Source: CAD feature listing. Evaluate the final solid. Frame: model axes, mm. Face numbers are marked on the shaded views. A direction names the side the tool comes from. Give positions to 0.01 mm unless a question says otherwise; leave off trailing zeros. Order: outer loops, then holes, each group sorted by start corner. A loop starts at its lowest first (then second) coordinate and runs counter-clockwise, first axis right, second up.
1) Section B-B, the plane z = -2.5. Return loops of the section in (x, y), plus the area to 3 significant figures.
2) Draft query along Z for the marked faces 1, 2 and 3. Return one class per face: released by +Z, released by -Z, zero draft, split by the parting line, or undercut.
3) Section D-D, the plane x = 27.5. Return loops of the section in (y, z).
4) First-contact query: P1, Ø2, axis at x = 79.5, z = -9, coming from the +Y side; P2, Ø8.5, axis at x = 86, z = -63.5, coming from the +Y side; P3, Ø5, axis at x = 48, y = 6, coming from the +Z side; P4, Ø2.5, axis at x = 2.5, z = -2.5, coming from the -Y side. Flat tips, straight axial feed; report the tip coordinate or a pass-through.
5) Material intervals for line 1 (Z direction, x = 2.5, y = 0.55); line 2 (X direction, y = 7.25, z = 7); line 3 (Z direction, x = 97.5, y = 1.15), sorted ascending.
6) Access query for the marked faces 4, 5, 6, 7 and 8. Directions: +Z, -Z, +X, -X, +Y, -Y. A direction counts if a zero-diameter tool reaches every point of the face in a straight line with its end or side. Return the directions, or none.
7) Section C-C, the plane z = -75. Return loops of the section in (x, y), plus the area to 3 significant figures.
8) Section A-A, the plane x = 55. Return loops of the section in (y, z), plus the area to 3 significant figures.
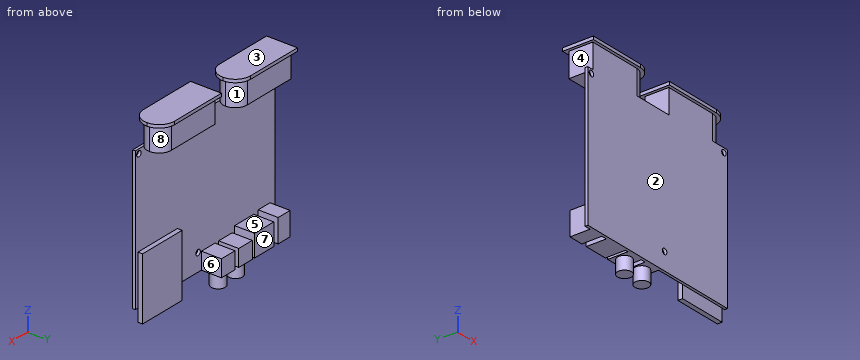
```python
from build123d import *

# Parameters (mm, degrees)
SKETCH1_W            = 100
SKETCH1_H            = 81
BOSS_EXTRUDE1_DEPTH  = 1.6
SKETCH2_W            = 38.5
SKETCH2_H            = 13.8
BOSS_EXTRUDE2_DEPTH  = 14
SKETCH3_W            = 42.4
SKETCH3_H            = 17.7
BOSS_EXTRUDE3_DEPTH  = 1.8
SKETCH4_W            = 8.5
SKETCH4_H            = 13.5
SKETCH4_W_2          = 13.7
SKETCH4_H_2          = 12.6
SKETCH4_W_3          = 9.7
SKETCH4_H_3          = 9.7
BOSS_EXTRUDE4_DEPTH  = 11.5
SKETCH5_W            = 28.3
SKETCH5_H            = 35.8
BOSS_EXTRUDE5_DEPTH  = 2.7
SKETCH6_R            = 4
BOSS_EXTRUDE6_DEPTH  = 7.5
M3_CLEARANCE_SLOT1_D = 3.2
FILLET1_R            = 7
FILLET2_R            = 8.8


with BuildPart() as part:
    # Sketch1 → Boss-Extrude1 (new body)
    with BuildSketch(Plane(origin=(0, 0, 0), x_dir=(1, 0, 0), z_dir=(0, 1, 0))):
        with Locations((50, 40.5)):
            Rectangle(SKETCH1_W, SKETCH1_H)
    extrude(amount=BOSS_EXTRUDE1_DEPTH)

    # Sketch2 → Boss-Extrude2 (add)
    with BuildSketch(Plane.XY):
        with Locations((77.25, 6.9)):
            Rectangle(SKETCH2_W, SKETCH2_H)
        with Locations((22.75, 6.9)):
            Rectangle(SKETCH2_W, SKETCH2_H)
    extrude(amount=BOSS_EXTRUDE2_DEPTH)

    # Sketch3 → Boss-Extrude3 (add)
    with BuildSketch(Plane.XY.offset(14)):
        with Locations((23, 7.15)):
            Rectangle(SKETCH3_W, SKETCH3_H)
        with Locations((77.5, 7.15)):
            Rectangle(SKETCH3_W, SKETCH3_H)
    extrude(amount=BOSS_EXTRUDE3_DEPTH)

    # Sketch4 → Boss-Extrude4 (add)
    with BuildSketch(Plane(origin=(0, 1.6, 0), x_dir=(1, 0, 0), z_dir=(0, 1, 0))):
        with Locations((7.706498822, 74.25)):
            Rectangle(SKETCH4_W, SKETCH4_H)
        with Locations((21.980965093, 74.7)):
            Rectangle(SKETCH4_W_2, SKETCH4_H_2)
        with Locations((35.395626501, 76.15)):
            Rectangle(SKETCH4_W_3, SKETCH4_H_3)
        with Locations((47.82718522, 76.15)):
            Rectangle(SKETCH4_W_3, SKETCH4_H_3)
    extrude(amount=BOSS_EXTRUDE4_DEPTH)

    # Sketch5 → Boss-Extrude5 (add)
    with BuildSketch(Plane(origin=(0, 1.6, 0), x_dir=(1, 0, 0), z_dir=(0, 1, 0))):
        with Locations((84.05, 70.3)):
            Rectangle(SKETCH5_W, SKETCH5_H)
    extrude(amount=BOSS_EXTRUDE5_DEPTH)

    # Sketch6 → Boss-Extrude6 (add)
    with BuildSketch(Plane(origin=(0, 0, -81), x_dir=(-1, 0, 0), z_dir=(0, 0, -1))):
        with Locations(Location((-47.82718522, 7.35, 0), (0, 0, 180))):
            Circle(SKETCH6_R)
        with Locations(Location((-35.395626501, 7.35, 0), (0, 0, 180))):
            Circle(SKETCH6_R)
    extrude(amount=BOSS_EXTRUDE6_DEPTH)

    # M3 Clearance Slot1 (through all)
    with Locations(Plane(origin=(0, 1.6, 0), x_dir=(1, 0, 0), z_dir=(0, 1, 0))):
        with Locations((55, 71), (97.5, 2.5), (2.5, 2.5)):
            Hole(M3_CLEARANCE_SLOT1_D / 2)

    # Fillet1
    # the kernel refuses this fillet: 7 mm, written as the material it takes off along each edge
    with BuildSketch(Plane(origin=(42, 0, 0), x_dir=(-1, 0, 0), z_dir=(0, 0, 1)), Plane(origin=(96.5, 0, 0), x_dir=(-1, 0, 0), z_dir=(0, 0, 1))) as fillet1_piece_1:
        with BuildLine():
            CenterArc((FILLET1_R, -FILLET1_R), FILLET1_R, 90, 90)
            Line((0, -FILLET1_R), (0, 0))
            Line((0, 0), (FILLET1_R, 0))
        make_face()
    extrude(amount=14, mode=Mode.SUBTRACT)
    with BuildSketch(Plane(origin=(42, 13.8, -17.5), x_dir=(0, -1, 0), z_dir=(0, 0, 1)), Plane(origin=(96.5, 13.8, -17.5), x_dir=(0, -1, 0), z_dir=(0, 0, 1))) as fillet1_piece_2:
        with BuildLine():
            CenterArc((FILLET1_R, -FILLET1_R), FILLET1_R, 90, 90)
            Line((0, -FILLET1_R), (0, 0))
            Line((0, 0), (FILLET1_R, 0))
        make_face()
    extrude(amount=31.5, mode=Mode.SUBTRACT)

    # Fillet2
    fillet2_edges = [part.edges().sort_by_distance(p)[0] for p in [
        (44.2, -1.7, 14.9),
        (44.2, 16, 14.9),
        (98.7, -1.7, 14.9),
        (98.7, 16, 14.9),
    ]]
    fillet(fillet2_edges, radius=FILLET2_R)


solid = part.part
```
From the geometry:
1. outline: (0, 0) - (0.9, 0) - (0.9, 1.6) - (0, 1.6) - close; (4.1, 0) - (95.9, 0) - (95.9, 1.6) - (4.1, 1.6) - close; (99.1, 0) - (100, 0) - (100, 1.6) - (99.1, 1.6) - close
1. area: 150 mm2
2. face 1: undercut
2. face 2: zero draft
2. face 3: released by +Z
3. outline: (-1.7, 14) - (0, 14) - (0, -81) - (13.1, -81) - (13.1, -68.4) - (1.6, -68.4) - (1.6, 0) - (13.8, 0) - (13.8, 14) - (16, 14) - (16, 15.8) - (-1.7, 15.8) - close
4. P1: stops at y = 1.6
4. P2: stops at y = 4.3
4. P3: stops at z = -71.3
4. P4: passes through
5. line 1: z = -81 to -4.1, -0.9 to 0, 14 to 15.8
5. line 2: x = 3.5 to 41.99, 58 to 96.49
5. line 3: z = -81 to -4.1, -0.9 to 0
6. face 4: -X, +Y, -Y
6. face 5: +Y
6. face 6: +Z, -Z, +Y
6. face 7: -Z, +X, -X, +Y
6. face 8: -Z, +X, +Y
7. outline: (0, 0) - (100, 0) - (100, 1.6) - (98.2, 1.6) - (98.2, 4.3) - (69.9, 4.3) - (69.9, 1.6) - (52.68, 1.6) - (52.68, 13.1) - (42.98, 13.1) - (42.98, 1.6) - (40.25, 1.6) - (40.25, 13.1) - (30.55, 13.1) - (30.55, 1.6) - (28.83, 1.6) - (28.83, 13.1) - (15.13, 13.1) - (15.13, 1.6) - (11.96, 1.6) - (11.96, 13.1) - (3.46, 13.1) - (3.46, 1.6) - (0, 1.6) - close
7. area: 715 mm2
8. outline: (0, -81) - (1.6, -81) - (1.6, -72.6) - (0, -72.6) - close; (0, -69.4) - (1.6, -69.4) - (1.6, 0) - (0, 0) - close
8. area: 124 mm2
